Part model, mm, in its own coordinate system. Face numbers are marked on the shaded views. A direction names the side the tool comes from. Give positions to 0.01 mm unless a question says otherwise; leave off trailing zeros. Write each loop counter-clockwise with the first axis right and the second up, starting at its lowest first coordinate (ties: lowest second). Pieces come first, ordered by that corner, then holes.
from build123d import *

# Parameters (mm, degrees)
SKETCH_2_R          = 2.6
CUT_EXTRUDE_1_DEPTH = 10


with BuildPart() as part:
    # 草图1 → 旋转1 (revolve)
    with BuildSketch(Plane(origin=(0, 0, 0), x_dir=(1, 0, 0), z_dir=(0, 1, 0))):
        Polygon((0, 0), (-5, 0), (-5, 9), (-11, 9), (-11, 14), (-22, 14), (-22, 16.4), (-11, 16.4), (-11, 54), (0, 54), align=None)
    revolve(axis=Axis((0, 0, -54), (0, 0, 1)))

    # 草图2 → 切除-拉伸1 (cut)
    with BuildSketch(Plane.XY.offset(-14)):
        with Locations((17.5, 0)):
            Circle(SKETCH_2_R)
        with Locations((-8.75, -15.155444566)):
            Circle(SKETCH_2_R)
        with Locations((-8.75, 15.155444566)):
            Circle(SKETCH_2_R)
    extrude(amount=-CUT_EXTRUDE_1_DEPTH, mode=Mode.SUBTRACT)


solid = part.part
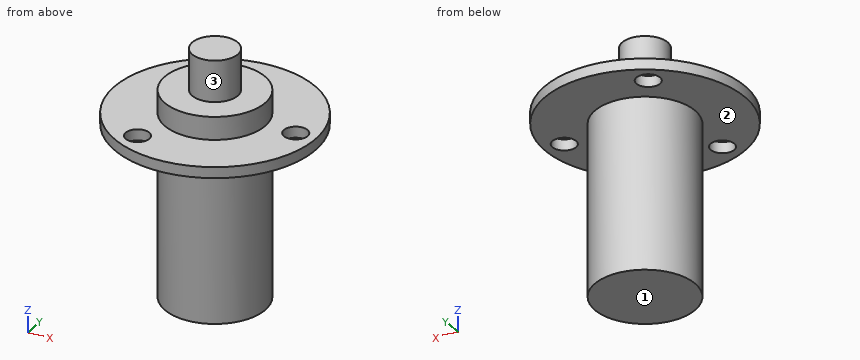
1) Saw through at C-C (x = 18). Write the cut outline in (y, z), and give its area (3 significant figures).
Check result:
outline: (-12.65, -16.4) - (-2.55, -16.4) - (-2.55, -14) - (-12.65, -14) - close; (2.55, -16.4) - (12.65, -16.4) - (12.65, -14) - (2.55, -14) - close
area: 48.5 mm2
2) Saw through at A-A (y = 0). Write the cut outline in (x, z).
Check result:
outline: (-22, -16.4) - (-11, -16.4) - (-11, -54) - (11, -54) - (11, -16.4) - (14.9, -16.4) - (14.9, -14) - (11, -14) - (11, -9) - (5, -9) - (5, 0) - (-5, 0) - (-5, -9) - (-11, -9) - (-11, -14) - (-22, -14) - close; (20.1, -16.4) - (22, -16.4) - (22, -14) - (20.1, -14) - close
3) 3-axis set-ups, long thin cutter, end or side, ignore diameter. For the marked faces 1, 2 and 3: which of +Z, -Z, +X, -X, +Y, -Y reach the whole face in a straight line?
Check result:
face 1: -Z, +X, -X, +Y, -Y
face 2: -Z
face 3: +Z
4) Flat gauge pins, fed straight in: P1, Ø8, axis at y = 0.5, z = -40.5, coming from the +X side; P2, Ø8, axis at x = 9.5, y = -2, coming from the +Z side; P3, Ø3, axis at x = -9, y = -11.5, coming from the -Z side; P4, Ø1.5, axis at x = -8.5, y = 14, coming from the -Z side. Where does each tip first touch, or does it go through?
Check result:
P1: stops at x = 11
P2: stops at z = -9
P3: stops at z = -16.4
P4: passes through
5) Saw through at B-B (x = 0). Write the cut outline in (y, z).
Check result:
outline: (-22, -16.4) - (-11, -16.4) - (-11, -54) - (11, -54) - (11, -16.4) - (22, -16.4) - (22, -14) - (11, -14) - (11, -9) - (5, -9) - (5, 0) - (-5, 0) - (-5, -9) - (-11, -9) - (-11, -14) - (-22, -14) - close
6) Saw through at D-D (z = -50). Write the cut outline in (x, y).
Check result:
outline: circle Ø22 at (0, 0)
7) Drill centre lines: L1, parallel to Y at x = -8.75, z = -15.05; L2, parallel to Z at x = -11.5, y = 17; L3, parallel to Y at x = 17.5, z = -15.6. Where is each one in solid material? Low to high.
Check result:
L1: y = -20.19 to -17.76, -12.56 to 12.56, 17.76 to 20.19
L2: z = -16.4 to -14
L3: y = -13.33 to -2.6, 2.6 to 13.33
